The drawing under review shows one solid part. Ordinate dimensions are in mm from its lowest x, y, z. A direction names the side the tool comes from. Round coordinates to 2 decimals unless told otherwise and drop trailing zeros. Order: outer loops, then holes, each group sorted by start corner. A loop starts at its lowest first (then second) coordinate and runs counter-clockwise, first axis right, second up.
1) Consider section B-B (z = 17.9). Give the boundary of the cut face in (x, y), then the cut area to 3 significant figures.
2) Clearance check with flat-ended pins moving along their axes: P1, Ø1, axis at x = 125, z = 17, coming from the +Y side; P2, Ø4, axis at x = 60, y = 16.5, coming from the +Z side; P3, Ø3.5, axis at x = 35, z = 17.9, coming from the -Y side. State where each tip first meets the part, or that it passes through.
3) Machinability: for the marked faces 1 and 2, which of the approach directions +Z, -Z, +X, -X, +Y, -Y give a long, thin tool a straight path to every point of the face, cutting with its end or side? Answer none if there is none.
4) Consider section A-A (x = 25). Give the boundary of the cut face in (y, z), then the cut area to 3 significant figures.
5) Consider section D-D (x = 136.5). Give the boundary of the cut face in (y, z), then the cut area to 3 significant figures.
6) To check wall thickness, follow L1, parallel to X at y = 3, z = 17.9; L2, parallel to Z at x = 115, y = 2.9; L3, parallel to Y at x = 125, z = 2.1. State the ranges of each line that lie inside material, in increasing order.
7) Consider section C-C (y = 12.5). Give the boundary of the cut face in (x, z).
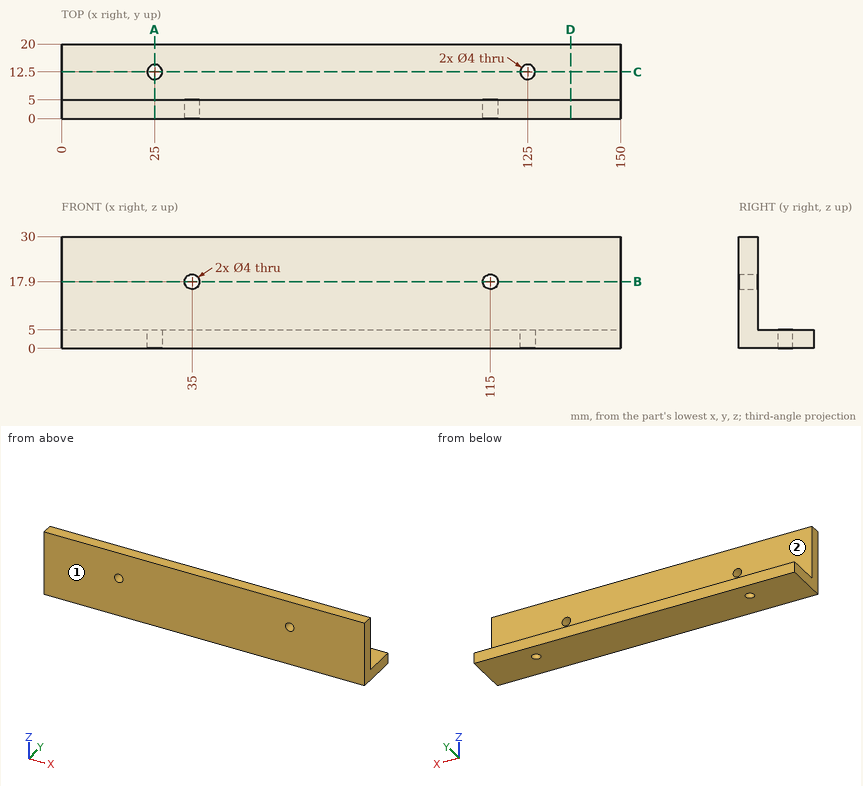
Answer below:
1. outline: (0, 0) - (33, 0) - (33, 5) - (0, 5) - close; (37, 0) - (113, 0) - (113, 5) - (37, 5) - close; (117, 0) - (150, 0) - (150, 5) - (117, 5) - close
1. area: 710 mm2
2. P1: stops at y = 5
2. P2: stops at z = 5
2. P3: passes through
3. face 1: +Z, -Z, +X, -X, -Y
3. face 2: +Z, +X, -X, +Y
4. outline: (0, 0) - (10.5, 0) - (10.5, 5) - (5, 5) - (5, 30) - (0, 30) - close; (14.5, 0) - (20, 0) - (20, 5) - (14.5, 5) - close
4. area: 205 mm2
5. outline: (0, 0) - (20, 0) - (20, 5) - (5, 5) - (5, 30) - (0, 30) - close
5. area: 225 mm2
6. L1: x = 0 to 33, 37 to 113, 117 to 150
6. L2: z = 0 to 15.9, 19.9 to 30
6. L3: y = 0 to 10.5, 14.5 to 20
7. outline: (0, 0) - (23, 0) - (23, 5) - (0, 5) - close; (27, 0) - (123, 0) - (123, 5) - (27, 5) - close; (127, 0) - (150, 0) - (150, 5) - (127, 5) - close
